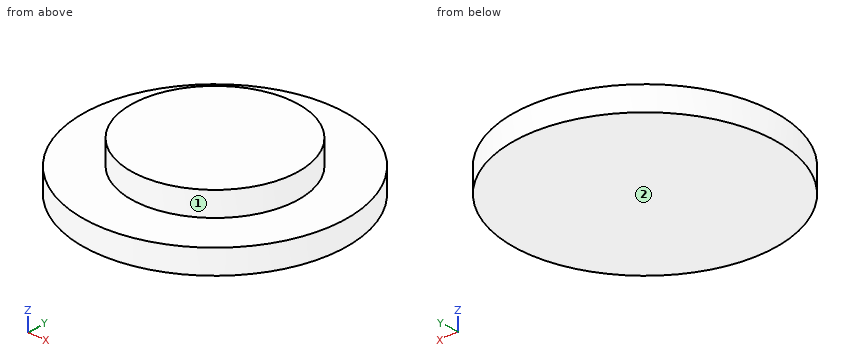
```python
from build123d import *

# Parameters (mm, degrees)
F0_R     = 34.322698
F1_DEPTH = 20
F2_R     = 53.945988
F3_DEPTH = 10
F4_R     = 45.735873
F5_DEPTH = 10


with BuildPart() as f1:
    # F0 (on Top) → F1 (new body)
    with BuildSketch(Plane.XY):
        Circle(F0_R)
    extrude(amount=F1_DEPTH)

    # F2 (on Top) → F3 (join)
    with BuildSketch(Plane.XY):
        Circle(F2_R)
    extrude(amount=F3_DEPTH)

    # F4 (on Top) → F5 (join)
    with BuildSketch(Plane.XY):
        Circle(F4_R)
    extrude(amount=F5_DEPTH)


solid = f1.part
```
Source: CAD feature listing. Evaluate the final solid. Frame: model axes, mm. Face numbers are marked on the shaded views. A direction names the side the tool comes from. Round coordinates to 2 decimals unless told otherwise and drop trailing zeros. Order: outer loops, then holes, each group sorted by start corner. A loop starts at its lowest first (then second) coordinate and runs counter-clockwise, first axis right, second up. Notation, with made-up numbers: (42, 41) -> (58, 41) arc R13 ccw to (58, 64) -> close; hole circle Ø7 at (-34, 38.5). An arc over 180 degrees is marked (long way). One line per item, written item: value. Start each with the question number.
Q1. Pin query (flat end, axial travel): pin 1 (10 mm diameter, centred on x = -31.5, z = 17.5, fed in from +Y); pin 2 (12 mm diameter, centred on x = -26, z = 17.5, fed in from -Y); pin 3 (1.5 mm diameter, centred on y = -4.5, z = 9, fed in from +X). Return the tip coordinate at first contact, or that it passes through.
Q2. Section query C-C (z = 16.5). Return the cut outline in (x, y), plus the area to 3 significant figures.
Q3. Material intervals for probe 1 along Z at (x, y) = (-36, -26.5); probe 2 along Y at (x, z) = (1.5, 9.75); probe 3 along Y at (x, z) = (45, 5.5), sorted ascending.
Q4. Section query D-D (z = 8.25). Return the cut outline in (x, y), plus the area to 3 significant figures.
Q5. Section query A-A (y = 0). Return the cut outline in (x, z), plus the area to 3 significant figures.
Q6. Access query for the marked faces 1 and 2. Directions: +Z, -Z, +X, -X, +Y, -Y. A direction counts if a zero-diameter tool reaches every point of the face in a straight line with its end or side. Return the directions, or none.
Findings below:
1. pin 1: y = 21.81
1. pin 2: y = -27.89
1. pin 3: x = 53.82
2. outline: circle Ø68.65 at (0, 0)
2. area: 3,700 mm²
3. probe 1: 0 to 10
3. probe 2: -53.93 to 53.93
3. probe 3: -29.75 to 29.75
4. outline: circle Ø107.89 at (0, 0)
4. area: 9,140 mm²
5. outline: (-53.95, 0) -> (53.95, 0) -> (53.95, 10) -> (34.32, 10) -> (34.32, 20) -> (-34.32, 20) -> (-34.32, 10) -> (-53.95, 10) -> close
5. area: 1,770 mm²
6. face 1: +Z
6. face 2: -Z, +X, -X, +Y, -Y
